from build123d import *

# Parameters (mm, degrees)
F0_R     = 1.85
F0_R_2   = 1.45
F0_R_3   = 1
F0_W     = 35
F0_H     = 50
F0_W_2   = 4
F0_H_2   = 10
F1_DEPTH = 2.5
F2_SIZE  = 2


# Not quite as in the source:
# - a feature names something its author has since deleted; it is built from what else it names


with BuildPart() as f1:
    # F0 (on Top) → F1 (new body)
    with BuildSketch(Plane.XY):
        Polygon((-12.5, 45), (-35, 45), (-35, -45), (35, -45), (35, 45), (12.5, 45), (12.5, 34), (-12.5, 34), align=None)
        with Locations((-30, -40)):
            Circle(F0_R, mode=Mode.SUBTRACT)
        with Locations((-22.5, -40)):
            Circle(F0_R_2, mode=Mode.SUBTRACT)
        with Locations((-11.5, -34)):
            Circle(F0_R_3, mode=Mode.SUBTRACT)
        with Locations((-30, -12.5)):
            Circle(F0_R_2, mode=Mode.SUBTRACT)
        with Locations((11.5, -34)):
            Circle(F0_R_3, mode=Mode.SUBTRACT)
        with Locations((22.5, -40)):
            Circle(F0_R_2, mode=Mode.SUBTRACT)
        with Locations((30, -40)):
            Circle(F0_R, mode=Mode.SUBTRACT)
        with Locations((0, -5)):
            Rectangle(F0_W, F0_H, mode=Mode.SUBTRACT)
        with Locations((30, -12.5)):
            Circle(F0_R_2, mode=Mode.SUBTRACT)
        with Locations((-22, 0)):
            Rectangle(F0_W_2, F0_H_2, mode=Mode.SUBTRACT)
        with Locations((-30, 12.5)):
            Circle(F0_R_2, mode=Mode.SUBTRACT)
        with Locations((-20, 40)):
            Circle(F0_R_2, mode=Mode.SUBTRACT)
        with Locations((-11.5, 24)):
            Circle(F0_R_3, mode=Mode.SUBTRACT)
        with Locations((22, 0)):
            Rectangle(F0_W_2, F0_H_2, mode=Mode.SUBTRACT)
        with Locations((30, 12.5)):
            Circle(F0_R_2, mode=Mode.SUBTRACT)
        with Locations((11.5, 24)):
            Circle(F0_R_3, mode=Mode.SUBTRACT)
        with Locations((20, 40)):
            Circle(F0_R_2, mode=Mode.SUBTRACT)
    extrude(amount=-F1_DEPTH)

    # F2
    f2_edges = [f1.edges().sort_by_distance(p)[0] for p in [
        (-35, -45, -1.25),
        (35, -45, -1.25),
    ]]
    chamfer(f2_edges, length=F2_SIZE)


solid = f1.part
Work out the finished part from the listing and answer in its coordinate system (mm). A direction names the side the tool comes from. Coordinates: 2 decimals unless noted, no trailing zeros. Loops run counter-clockwise (first coordinate to the right, second up) from the corner with the lowest first, then second, coordinate; pieces in that order, holes last. Notation, with made-up numbers: (69.25, -33) -> (74.25, -33) arc R20 cw to (74.25, -17) -> close; hole circle Ø10 at (45.5, 7). An arc over 180 degrees is marked (long way). Write each question's results on one line, items separated by ' | '. Start each with the question number.
1) Consider line 1 along X through (y, z) = (0, -0.3); line 2 along Y through (x, z) = (22.5, -0.85); line 3 along Y through (x, z) = (-30, -1.1). Determine where each line is inside the solid, lowest interval first.
2) For faces 1 (the flat face through (22, -5, -1)), 2 (the flat face through (-12.5, 39, -1)), 3 (the flat face through (35, 0, -1)), determine the directions among +Z, -Z, +X, -X, +Y, -Y from which every point of the face is accessible in a straight line to the end or side of a thin tool.
3) The mould has two halves that part along Y. Classify faces 4 (the flat face through (-17.5, -5, -1)), 5 (the flat face through (0, 21, -2.5)), 6 (the flat face through (0, -45, -1)), 7 (the cylindrical face through (-18.661, 39.445, -1.232)): pulls with the +Y half, pulls with the -Y half, needs draft (parallel to the pull), parting line crosses it, or undercut.
4) Flat-ended cylindrical pins translate along their axes: P1, Ø3.5, axis at x = 30, y = 12.5, coming from the -Z side; P2, Ø1.2, axis at x = -11.5, y = 24, coming from the +Z side. Find the tip coordinate at first contact, or state that the pin passes through.
5) Find section A-A on x = 5. Determine the outline of the cut face in (y, z), then the cut area to 3 significant figures.
6) Find section D-D on y = -25. Determine the outline of the cut face in (x, z).
7) Find section C-C on x = -11.5. Determine the outline of the cut face in (y, z).
8) Find section B-B on y = -40. Determine the outline of the cut face in (x, z), then the cut area to 3 significant figures.
Response values:
1) line 1: x = -35 to -24, -20 to -17.5, 17.5 to 20, 24 to 35 | line 2: y = -45 to -41.45, -38.55 to -5, 5 to 45 | line 3: y = -45 to -41.85, -38.15 to -13.95, -11.05 to 11.05, 13.95 to 45
2) face 1: +Z, -Z | face 2: +Z, -Z, +Y | face 3: +Z, -Z, +X, +Y, -Y
3) face 4: undercut | face 5: needs draft | face 6: pulls with the -Y half | face 7: undercut
4) P1: stops at z = -2.5 | P2: passes through
5) outline: (-45, -2.5) -> (-30, -2.5) -> (-30, 0) -> (-45, 0) -> close; (20, -2.5) -> (34, -2.5) -> (34, 0) -> (20, 0) -> close | area: 72.5 mm^2
6) outline: (-35, -2.5) -> (-17.5, -2.5) -> (-17.5, 0) -> (-35, 0) -> close; (17.5, -2.5) -> (35, -2.5) -> (35, 0) -> (17.5, 0) -> close
7) outline: (-45, -2.5) -> (-35, -2.5) -> (-35, 0) -> (-45, 0) -> close; (-33, -2.5) -> (-30, -2.5) -> (-30, 0) -> (-33, 0) -> close; (20, -2.5) -> (23, -2.5) -> (23, 0) -> (20, 0) -> close; (25, -2.5) -> (34, -2.5) -> (34, 0) -> (25, 0) -> close
8) outline: (-35, -2.5) -> (-31.85, -2.5) -> (-31.85, 0) -> (-35, 0) -> close; (-28.15, -2.5) -> (-23.95, -2.5) -> (-23.95, 0) -> (-28.15, 0) -> close; (-21.05, -2.5) -> (21.05, -2.5) -> (21.05, 0) -> (-21.05, 0) -> close; (23.95, -2.5) -> (28.15, -2.5) -> (28.15, 0) -> (23.95, 0) -> close; (31.85, -2.5) -> (35, -2.5) -> (35, 0) -> (31.85, 0) -> close | area: 142 mm^2
